CAD build for the part. Positions are in the model's coordinates, mm. Face numbers are marked on the shaded views. A direction names the side the tool comes from. Round coordinates to 2 decimals unless told otherwise and drop trailing zeros. Order: outer loops, then holes, each group sorted by start corner. A loop starts at its lowest first (then second) coordinate and runs counter-clockwise, first axis right, second up. Notation, with made-up numbers: M 29.25,-13.75 L 37.25,-13.75 A21 ccw 37.25,5.25 Z; hole C 55.5,27 d9. An arc over 180 degrees is marked long. Answer as a JSON object with one key per item and string values.
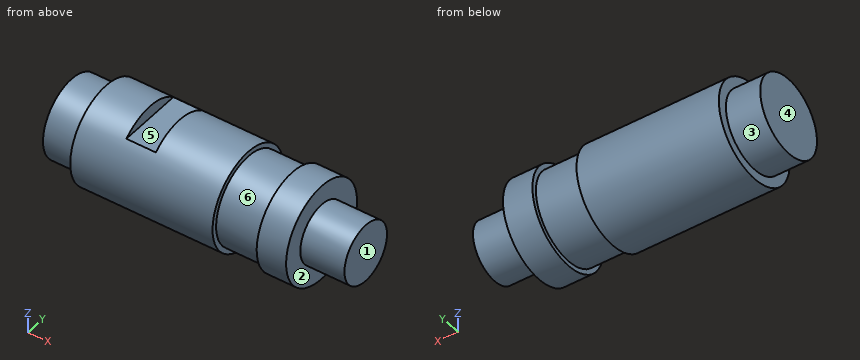
```python
from build123d import *

# Parameters (mm, degrees)
F0_W     = 11.1125
F0_H     = 12.7
F0_W_2   = 14.2875
F0_H_2   = 14.2875
F0_H_3   = 9.525
F2_W     = 9.5377
F2_H     = 23.704022
F3_DEPTH = 63.5


with BuildPart() as f1:
    # F0 (on Front) → F1 (revolve)
    with BuildSketch(Plane.XZ):
        with Locations((-42.06875, 6.35)):
            Rectangle(F0_W, F0_H)
        Polygon((-36.5125, 12.7), (-36.5125, 0), (9.5377, 0), (9.5377, 14.2875), (9.5377, 15.875), (-36.5125, 15.875), align=None)
        with Locations((16.68145, 7.14375)):
            Rectangle(F0_W_2, F0_H_2)
        Polygon((23.8252, 14.2875), (23.8252, 0), (33.3375, 0), (33.3375, 9.525), (33.3375, 15.875), (23.8125, 15.875), align=None)
        with Locations((40.48125, 4.7625)):
            Rectangle(F0_W_2, F0_H_3)
    revolve(axis=Axis((0, 0, 0), (1, 0, 0)))

    # F2 (on Front) → F3 (cut, symmetric)
    with BuildSketch(Plane.XZ):
        with Locations((-17.45615, 23.758261)):
            Rectangle(F2_W, F2_H)
    extrude(amount=F3_DEPTH, both=True, mode=Mode.SUBTRACT)


solid = f1.part
```
Item 1: Saw through at B-B on y = 0. List the corners of the cut face in (x, z) (1 decimal), and give its area (3 significant figures).
Worked answers:
{"outline": "M -47.6,-12.7 L -36.5,-12.7 L -36.5,-15.9 L 9.5,-15.9 L 9.5,-14.3 L 23.8,-14.3 L 23.8,-15.9 L 33.3,-15.9 L 33.3,-9.5 L 47.6,-9.5 L 47.6,9.5 L 33.3,9.5 L 33.3,15.9 L 23.8,15.9 L 23.8,14.3 L 9.5,14.3 L 9.5,15.9 L -12.7,15.9 L -12.7,11.9 L -22.2,11.9 L -22.2,15.9 L -36.5,15.9 L -36.5,12.7 L -47.6,12.7 Z", "area": "2,690 mm2"}
Item 2: Saw through at D-D on x = -20. List the corners of the cut face in (y, z) (3 decimals).
Worked answers:
{"outline": "M -10.5,11.906 A15.875 ccw long 10.5,11.906 Z"}
Item 3: 3-axis set-ups, long thin cutter, end or side, ignore diameter. For the marked faces 1 and 2: which of +Z, -Z, +X, -X, +Y, -Y reach the whole face in a straight line?
Worked answers:
{"face 1": "+Z, -Z, +X, +Y, -Y", "face 2": "+X"}
Item 4: Drop flat-ended pins along their axis: pin 1 Ø2 at (y, z) = (12, 9.5) entering from +X; pin 2 Ø1.5 at (x, y) = (37.5, 7) entering from +Z; pin 3 Ø6 at (x, y) = (-4, -5.5) entering from -Z. Give the stop position or say it passes through.
Worked answers:
{"pin 1": "stops at x = 33.34", "pin 2": "stops at z = 7.19", "pin 3": "stops at z = -15.68"}
Item 5: Saw through at A-A on z = 0. List the corners of the cut face in (x, y) (1 decimal), and give its area (3 significant figures).
Worked answers:
{"outline": "M -47.6,-12.7 L -36.5,-12.7 L -36.5,-15.9 L 9.5,-15.9 L 9.5,-14.3 L 23.8,-14.3 L 23.8,-15.9 L 33.3,-15.9 L 33.3,-9.5 L 47.6,-9.5 L 47.6,9.5 L 33.3,9.5 L 33.3,15.9 L 23.8,15.9 L 23.8,14.3 L 9.5,14.3 L 9.5,15.9 L -36.5,15.9 L -36.5,12.7 L -47.6,12.7 Z", "area": "2,730 mm2"}
Item 6: Two-plate mould, pull along X, no slides. Class the marked faces 3, 4, 5 and 6: released by +X, released by -X, zero draft, split by the parting line, or undercut.
Worked answers:
{"face 3": "zero draft", "face 4": "released by -X", "face 5": "undercut", "face 6": "undercut"}
Item 7: Wall check: line 1 along X through (y, z) = (-9, 13) (1 decimal); line 2 along X through (y, z) = (10, -12); line 3 along X through (y, z) = (-0.5, 12) (1 decimal). Give the ranges that are in metal, low to high. Write a range as [from, to].
Worked answers:
{"line 1": "x = [-36.5, -22.2], [-12.7, 9.5], [23.8, 33.3]", "line 2": "x = [-36.51, 9.54], [23.81, 33.34]", "line 3": "x = [-47.6, -22.2], [-12.7, 33.3]"}
Item 8: Saw through at C-C on x = 40. List the corners of the cut face in (y, z) (3 decimals), and give its area (3 significant figures).
Worked answers:
{"outline": "C 0,0 d19.05", "area": "285 mm2"}
